Source: CAD feature listing. Evaluate the final solid. Frame: model axes, mm. A direction names the side the tool comes from. Give positions to 0.01 mm unless a question says otherwise; leave off trailing zeros. Write each loop counter-clockwise with the first axis right and the second up, starting at its lowest first coordinate (ties: lowest second). Pieces come first, ordered by that corner, then holes. Notation, with made-up numbers: (41.25, -36) - (79.25, -36) arc R21 cw to (79.25, 1) - close; hole circle Ø11 at (17, 19.5). An arc over 180 degrees is marked (long way). One line per question, with ' | ' between items. Start each with the question number.
(1) Section C-C, the plane x = 91.5. Return loops of the section in (y, z).
(2) Section A-A, the plane x = 11. Return loops of the section in (y, z), plus the area to 3 significant figures.
(3) Access query for faces 4 (the cylindrical face through (104.084, 0.358, -32.523)), 5 (the cylindrical face through (1.01, -23.3, -3.06)), 6 (the flat face through (71, 15, 30)), 7 (the cylindrical face through (77.902, 68.335, -15.175)). Directions: +Z, -Z, +X, -X, +Y, -Y. A direction counts if a zero-diameter tool reaches every point of the face in a straight line with its end or side. Return the directions, or none.
(4) Section B-B, the plane z = -49.5. Return loops of the section in (x, y).
(5) Pin query (flat end, axial travel): pin 1 (16 mm diameter, centred on y = 28.55, z = 49.44, fed in from -X); pin 2 (3 mm diameter, centred on x = 28.5, y = 7.5, fed in from +Z); pin 3 (10 mm diameter, centred on x = 17.5, z = -27.5, fed in from -Y). Return the tip coordinate at first contact, or that it passes through.
(6) Draft query along Y for faces 1 (the cylindrical face through (11.496, 34.168, -7.587)), 2 (the flat face through (17.85, -19, 7)), 3 (the flat face through (0, 23, 7)). Return one class per face: +Y half, -Y half, draft (parallel to the pull), parting line (faces both ways), or undercut.
(7) Ray query, line 1 (Y direction, x = 102.5, z = 0); line 2 (Y direction, x = 3.4, z = 0); line 3 (Y direction, x = 7.5, z = 0). Return the intervals inside material, ascending. Write a range as [from, to].
```python
from build123d import *

# Parameters (mm, degrees)
FORO_12_5_12_5_1_D          = 12.5
RIPETIZIONECIRCOLARE1_COUNT = 6
RIPETIZIONECIRCOLARE2_COUNT = 4


with BuildPart() as part:
    # Schizzo1 → Rivoluzione1 (revolve)
    with BuildSketch(Plane.XY, mode=Mode.PRIVATE) as rivoluzione1_sk:
        Polygon((0, 35), (0, 23.5), (2, 23.5), (2, 24.75), (3.85, 24.75), (3.85, 23.5), (17.85, 23.5), (17.85, 20), (94.5, 20), (94.5, 26), (110, 26), (110, 45.5), (85, 45.5), (85, 70), (71, 70), (71, 30), (28.317889407, 30), (23.317889407, 35), align=None)
    revolve(rivoluzione1_sk.sketch.rotate(Axis((-28.748065329, 0, 0), (1, 0, 0)), 90), axis=Axis((-28.748065329, 0, 0), (1, 0, 0)))

    # Foro Ø12.5 (12.5)-1 (through all)
    with Locations(Plane.ZY.offset(-71)):
        with Locations((0, 57.09)):
            foro_12_5_12_5_1 = Hole(FORO_12_5_12_5_1_D / 2)

    # RipetizioneCircolare1: Foro Ø12.5 (12.5)-1 ×6 about axis
    ripetizionecircolare1_axis = Axis((0, 0, 0), (1, 0, 0))
    for i in range(1, RIPETIZIONECIRCOLARE1_COUNT):
        add(foro_12_5_12_5_1.rotate(ripetizionecircolare1_axis, i * 360 / RIPETIZIONECIRCOLARE1_COUNT), mode=Mode.SUBTRACT)

    # Schizzo7 → Foro per Vite M5-1 (revolve, cut)
    with BuildSketch(Plane(origin=(110, 35.25, 0), x_dir=(0, 0, -1), z_dir=(0, 1, 0))):
        Polygon((0, 0), (0, 13.652366702), (2.75, 12), (2.75, 0), align=None)
    foro_per_vite_m5_1 = revolve(axis=Axis((116.35, 35.25, 0), (-1, 0, 0)), mode=Mode.SUBTRACT)

    # RipetizioneCircolare2: Foro per Vite M5-1 ×4 about axis
    ripetizionecircolare2_axis = Axis((0, 0, 0), (1, 0, 0))
    for i in range(1, RIPETIZIONECIRCOLARE2_COUNT):
        add(foro_per_vite_m5_1.rotate(ripetizionecircolare2_axis, i * 360 / RIPETIZIONECIRCOLARE2_COUNT), mode=Mode.SUBTRACT)


solid = part.part
```
Check sheet entries:
1) outline: circle Ø91 at (0, 0); hole circle Ø40 at (0, 0)
2) outline: circle Ø70 at (0, 0); hole circle Ø47 at (0, 0) | area: 2,110 mm²
3) face 4: +X | face 5: -X | face 6: none | face 7: +X, -X
4) outline: (71, -49.49) - (85, -49.49) - (85, -34.79) - (71, -34.79) - close; (71, -22.3) - (85, -22.3) - (85, 22.3) - (71, 22.3) - close; (71, 34.79) - (85, 34.79) - (85, 49.49) - (71, 49.49) - close
5) pin 1: x = 71 | pin 2: z = 30.45 | pin 3: y = -26.81
6) face 1: parting line | face 2: undercut | face 3: draft
7) line 1: [-45.5, -38], [-32.5, -26], [26, 32.5], [38, 45.5] | line 2: [-35, -24.75], [24.75, 35] | line 3: [-35, -23.5], [23.5, 35]
